Geometry check sheet. Reference: the model listing, model coordinates, mm. A direction names the side the tool comes from. Round coordinates to 2 decimals unless told otherwise and drop trailing zeros. Write each loop counter-clockwise with the first axis right and the second up, starting at its lowest first coordinate (ties: lowest second). Pieces come first, ordered by that corner, then holes. Notation, with made-up numbers: M 19,32 L 70,32 A17 cw 70,52 Z; hole C -6.5,4.5 d10. An arc over 180 degrees is marked long. Use a Markdown table: item, result.
Autodesk Inventor part; units mm, degrees
ref_plane "YZ Plane" through (0, 0, 0) normal (1, 0, 0) x (0, 1, 0)
ref_plane "XZ Plane" through (0, 0, 0) normal (0, 1, 0) x (-1, 0, 0)
ref_plane "XY Plane" through (0, 0, 0) normal (0, 0, 1) x (1, 0, 0)
sketch "Szkic1" plane through (0, 0, 0) normal (0, 0, 1) x (1, 0, 0)
  arc A0 (-1.732, -4.0613) -> (-1.6613, -4.132) centre (0, -2.4) ccw
  arc A1 (0.05, -0.4006) -> (-0.05, -0.4006) centre (0, -2.4) ccw
  arc A2 (-0.05, -0.4006) -> (-0.5703, -0.483) centre (0, -2.4) ccw
  arc A3 (-0.5703, -0.483) -> (-0.6654, -0.5139) centre (0, -2.4) ccw
  arc A4 (-0.6654, -0.5139) -> (-1.1348, -0.7531) centre (0, -2.4) ccw
  arc A5 (-1.1348, -0.7531) -> (-1.2157, -0.8119) centre (0, -2.4) ccw
  arc A6 (-1.2157, -0.8119) -> (-1.5881, -1.1843) centre (0, -2.4) ccw
  arc A7 (-1.5881, -1.1843) -> (-1.6469, -1.2652) centre (0, -2.4) ccw
  arc A8 (-1.6469, -1.2652) -> (-1.8861, -1.7346) centre (0, -2.4) ccw
  arc A9 (-1.8861, -1.7346) -> (-1.917, -1.8297) centre (0, -2.4) ccw
  arc A10 (-1.917, -1.8297) -> (-1.9994, -2.35) centre (0, -2.4) ccw
  arc A11 (-1.9994, -2.35) -> (-1.9994, -2.45) centre (0, -2.4) ccw
  arc A12 (-1.9994, -2.45) -> (-1.917, -2.9703) centre (0, -2.4) ccw
  arc A13 (-1.917, -2.9703) -> (-1.8861, -3.0654) centre (0, -2.4) ccw
  arc A14 (-1.8861, -3.0654) -> (-1.6469, -3.5348) centre (0, -2.4) ccw
  arc A15 (-1.6469, -3.5348) -> (-1.5881, -3.6157) centre (0, -2.4) ccw
  arc A16 (-1.5881, -3.6157) -> (-1.2157, -3.9881) centre (0, -2.4) ccw
  arc A17 (-1.2157, -3.9881) -> (-1.1348, -4.0469) centre (0, -2.4) ccw
  arc A18 (-1.1348, -4.0469) -> (-0.6654, -4.2861) centre (0, -2.4) ccw
  arc A19 (-0.6654, -4.2861) -> (-0.5703, -4.317) centre (0, -2.4) ccw
  arc A20 (-0.5703, -4.317) -> (-0.05, -4.3994) centre (0, -2.4) ccw
  arc A21 (-0.05, -4.3994) -> (0.05, -4.3994) centre (0, -2.4) ccw
  arc A22 (0.05, -4.3994) -> (0.5703, -4.317) centre (0, -2.4) ccw
  arc A23 (0.5703, -4.317) -> (0.6654, -4.2861) centre (0, -2.4) ccw
  arc A24 (0.6654, -4.2861) -> (1.1348, -4.0469) centre (0, -2.4) ccw
  arc A25 (1.1348, -4.0469) -> (1.2157, -3.9881) centre (0, -2.4) ccw
  arc A26 (1.2157, -3.9881) -> (1.5881, -3.6157) centre (0, -2.4) ccw
  arc A27 (1.5881, -3.6157) -> (1.6469, -3.5348) centre (0, -2.4) ccw
  arc A28 (1.6469, -3.5348) -> (1.8861, -3.0654) centre (0, -2.4) ccw
  arc A29 (1.8861, -3.0654) -> (1.917, -2.9703) centre (0, -2.4) ccw
  arc A30 (1.917, -2.9703) -> (1.9994, -2.45) centre (0, -2.4) ccw
  arc A31 (1.9994, -2.45) -> (1.9994, -2.35) centre (0, -2.4) ccw
  arc A32 (1.9994, -2.35) -> (1.917, -1.8297) centre (0, -2.4) ccw
  arc A33 (1.917, -1.8297) -> (1.8861, -1.7346) centre (0, -2.4) ccw
  arc A34 (1.8861, -1.7346) -> (1.6469, -1.2652) centre (0, -2.4) ccw
  arc A35 (1.6469, -1.2652) -> (1.5881, -1.1843) centre (0, -2.4) ccw
  arc A36 (1.5881, -1.1843) -> (1.2157, -0.8119) centre (0, -2.4) ccw
  arc A37 (1.2157, -0.8119) -> (1.1348, -0.7531) centre (0, -2.4) ccw
  arc A38 (1.1348, -0.7531) -> (0.6654, -0.5139) centre (0, -2.4) ccw
  arc A39 (0.6654, -0.5139) -> (0.5703, -0.483) centre (0, -2.4) ccw
  arc A40 (0.5703, -0.483) -> (0.05, -0.4006) centre (0, -2.4) ccw
  circle A41 centre (0, -2.4) radius 1.5065
  circle A42 centre (0, -2.4) radius 2.4
  circle A43 centre (0, -2.4) radius 15
  circle A44 centre (0, -2.4) radius 1.0065
  circle A45 centre (0, -2.4) radius 1.2565
  circle A46 centre (0, -2.4) radius 2.9
  point P0 (0, 0)
  point P1 (-1.6613, -4.132)
  point P2 (-1.732, -4.0613)
  dimension "d0" = 30
  dimension "d3" = 0.25
  dimension "d12" = 0.5
extrude "Wyciągnięcie proste1" add sketch "Szkic1" against normal blind 3 contours A43
extrude "Wyciągnięcie proste2" add sketch "Szkic1" along normal blind 1.5 contours A42 A0 | A40 A39 A38 A37 A36 A35 A34 A33 A32 A31 A30 A29 A28 A27 A26 A25 A24 A23 A22 A21 A20 A19 A18 A17 A16 A15 A14 A13 A12 A11 A10 A9 A8 A7 A6 A5 A4 A3 A2 A1 | A41 | A43 | A45 | A46
sketch "Szkic2" plane through (0, -2.4, 1.5) normal (0, 0, 1) x (1, 0, 0)
  circle A0 centre (0, 0) radius 1.0065
  circle A1 centre (0, 0) radius 3
  circle A2 centre (0, 0) radius 15
  point P0 (0, 2.4)
  dimension "d6" = 6
extrude "Wyciągnięcie proste3" add sketch "Szkic2" along normal blind 2.7 contours A2
sketch "Szkic4" plane through (0, -2.4, -3) normal (0, 0, -1) x (-1, 0, 0)
  arc A0 (6.703, -7.1797) -> (6.021, -7.7605) centre (12.6436, -14.8459) ccw
  arc A1 (9.8735, -5.5514) -> (9.0277, -5.8466) centre (12.6436, -14.8459) ccw
  arc A2 (13.4181, -5.1783) -> (12.5228, -5.1481) centre (12.6436, -14.8459) ccw
  arc A3 (16.8582, -6.1109) -> (16.0342, -5.7593) centre (12.6436, -14.8459) ccw
  arc A4 (19.729, -8.2232) -> (19.0877, -7.5977) centre (12.6436, -14.8459) ccw
  arc A5 (21.6429, -11.23) -> (21.2709, -10.4151) centre (12.6436, -14.8459) ccw
  arc A6 (22.3415, -14.7251) -> (22.2889, -13.8308) centre (12.6436, -14.8459) ccw
  arc A7 (21.7302, -18.2365) -> (22.0043, -17.3836) centre (12.6436, -14.8459) ccw
  arc A8 (19.8918, -21.29) -> (20.4555, -20.5937) centre (12.6436, -14.8459) ccw
  arc A9 (3.9087, -10.6314) -> (5.6223, -12.2259) centre (9.734, -6.0892) ccw
  arc A10 (5.6223, -12.2259) -> (5.4105, -12.8849) centre (12.6436, -14.8459) ccw
  arc A11 (5.4105, -12.8849) -> (3.0888, -13.1827) centre (5.1774, -20.2681) ccw
  arc A12 (3.0888, -13.1827) -> (2.9761, -14.0714) centre (12.6436, -14.8459) ccw
  arc A13 (2.9761, -14.0714) -> (5.1499, -14.9393) centre (6.7672, -7.7316) ccw
  arc A14 (5.1499, -14.9393) -> (5.1905, -15.6303) centre (12.6436, -14.8459) ccw
  arc A15 (5.1905, -15.6303) -> (3.1332, -16.7466) centre (7.6403, -22.5991) ccw
  arc A16 (3.1332, -16.7466) -> (3.3491, -17.616) centre (12.6436, -14.8459) ccw
  arc A17 (3.3491, -17.616) -> (5.6897, -17.64) centre (4.594, -10.3348) ccw
  arc A18 (5.6897, -17.64) -> (5.9772, -18.2697) centre (12.6436, -14.8459) ccw
  arc A19 (5.9772, -18.2697) -> (4.462, -20.0539) centre (10.7789, -23.883) ccw
  arc A20 (4.462, -20.0539) -> (4.9774, -20.7866) centre (12.6436, -14.8459) ccw
  arc A21 (4.9774, -20.7866) -> (7.1686, -19.9634) centre (3.508, -13.5473) ccw
  arc A22 (7.1686, -19.9634) -> (7.6642, -20.4467) centre (12.6436, -14.8459) ccw
  arc A23 (7.6642, -20.4467) -> (6.8958, -22.6577) centre (14.1694, -23.9463) ccw
  arc A24 (6.8958, -22.6577) -> (7.6411, -23.1547) centre (12.6436, -14.8459) ccw
  arc A25 (7.6411, -23.1547) -> (9.387, -21.5956) centre (3.6558, -16.9352) ccw
  arc A26 (9.387, -21.5956) -> (10.0237, -21.8673) centre (12.6436, -14.8459) ccw
  arc A27 (10.0237, -21.8673) -> (10.1059, -24.2066) centre (17.3539, -22.7806) ccw
  arc A28 (10.1059, -24.2066) -> (10.9804, -24.4008) centre (12.6436, -14.8459) ccw
  arc A29 (10.9804, -24.4008) -> (12.0452, -22.3162) centre (5.0175, -20.0409) ccw
  arc A30 (12.0452, -22.3162) -> (12.737, -22.3396) centre (12.6436, -14.8459) ccw
  arc A31 (12.737, -22.3396) -> (13.6588, -24.4912) centre (19.9021, -20.5433) ccw
  arc A32 (13.6588, -24.4912) -> (14.5444, -24.3564) centre (12.6436, -14.8459) ccw
  arc A33 (14.5444, -24.3564) -> (14.7842, -22.028) centre (7.4091, -22.4449) ccw
  arc A34 (14.7842, -22.028) -> (15.4377, -21.7998) centre (12.6436, -14.8459) ccw
  arc A35 (15.4377, -21.7998) -> (17.0745, -23.4732) centre (21.4701, -17.5365) ccw
  arc A36 (17.0745, -23.4732) -> (17.8516, -23.0275) centre (12.6436, -14.8459) ccw
  arc A37 (17.8516, -23.0275) -> (17.2341, -20.7697) centre (10.5077, -23.8227) ccw
  arc A38 (17.2341, -20.7697) -> (17.7611, -20.3209) centre (12.6436, -14.8459) ccw
  arc A39 (17.7611, -20.3209) -> (19.8918, -21.29) centre (21.846, -14.1663) ccw
  arc A40 (20.4555, -20.5937) -> (19.0641, -18.7114) centre (13.8947, -23.9881) ccw
  arc A41 (19.0641, -18.7114) -> (19.3933, -18.1026) centre (12.6436, -14.8459) ccw
  arc A42 (19.3933, -18.1026) -> (21.7302, -18.2365) centre (20.9791, -10.8879) ccw
  arc A43 (22.0043, -17.3836) -> (20.0269, -16.1311) centre (17.1128, -22.9188) ccw
  arc A44 (20.0269, -16.1311) -> (20.114, -15.4444) centre (12.6436, -14.8459) ccw
  arc A45 (20.114, -15.4444) -> (22.3415, -14.7251) centre (18.9865, -8.1441) ccw
  arc A46 (22.2889, -13.8308) -> (19.9926, -13.3772) centre (19.7273, -20.7593) ccw
  arc A47 (19.9926, -13.3772) -> (19.8257, -12.7054) centre (12.6436, -14.8459) ccw
  arc A48 (19.8257, -12.7054) -> (21.6429, -11.23) centre (16.1372, -6.3053) ccw
  arc A49 (21.2709, -10.4151) -> (18.9658, -10.8216) centre (21.3851, -17.801) ccw
  arc A50 (18.9658, -10.8216) -> (18.5675, -10.2554) centre (12.6436, -14.8459) ccw
  arc A51 (18.5675, -10.2554) -> (19.729, -8.2232) centre (12.816, -5.6201) ccw
  arc A52 (19.0877, -7.5977) -> (17.0851, -8.8095) centre (21.8623, -14.4437) ccw
  arc A53 (17.0851, -8.8095) -> (16.5092, -8.4255) centre (12.6436, -14.8459) ccw
  arc A54 (16.5092, -8.4255) -> (16.8582, -6.1109) centre (9.4716, -6.1808) ccw
  arc A55 (16.0342, -5.7593) -> (14.6046, -7.6127) centre (21.0945, -11.1407) ccw
  arc A56 (14.6046, -7.6127) -> (13.9288, -7.4626) centre (12.6436, -14.8459) ccw
  arc A57 (13.9288, -7.4626) -> (13.4181, -5.1783) centre (6.5556, -7.9118) ccw
  arc A58 (12.5228, -5.1481) -> (11.8593, -7.3928) centre (19.1854, -8.3381) ccw
  arc A59 (11.8593, -7.3928) -> (11.1749, -7.4969) centre (12.6436, -14.8459) ccw
  arc A60 (11.1749, -7.4969) -> (9.8735, -5.5514) centre (4.4619, -10.5793) ccw
  arc A61 (9.0277, -5.8466) -> (9.2198, -8.1794) centre (16.3927, -6.4144) ccw
  arc A62 (9.2198, -8.1794) -> (8.6193, -8.5238) centre (12.6436, -14.8459) ccw
  arc A63 (8.6193, -8.5238) -> (6.703, -7.1797) centre (3.4731, -13.823) ccw
  arc A64 (6.021, -7.7605) -> (7.0428, -9.8664) centre (13.0938, -5.6294) ccw
  arc A65 (7.0428, -9.8664) -> (6.6073, -10.4044) centre (12.6436, -14.8459) ccw
  arc A66 (6.6073, -10.4044) -> (4.3348, -9.8434) centre (3.7228, -17.2049) ccw
  arc A67 (4.3348, -9.8434) -> (3.9087, -10.6314) centre (12.6436, -14.8459) ccw
  point P0 (0, 2.4)
  point P1 (0, 0)
extrude "Wyciągnięcie proste5" cut sketch "Szkic4" against normal blind 10 keep common part
properties part number "small-gear"
Item 1: Material ranges on line 1 along Y through (x, z) = (-6.75, -2.5); line 2 along Y through (x, z) = (-6.25, 2.75); line 3 along X through (y, z) = (-9.25, 1.5), recorded low to high. Write a range as from..to.
Outcome:
| item | result |
|---|---|
| line 1 | y = -15.8..-12.62, -11.81..-9.6 |
| line 2 | y = -16.04..-12.66, -10.81..-9.95 |
| line 3 | x = -13.34..-11.95, -10.84..-9.02 |
Item 2: Cross-section at C-C, the plane x = -8. Record the cut outline in (y, z), and give its area (3 significant figures).
Outcome:
| item | result |
|---|---|
| outline | M -15.09,-3 L -10.39,-3 L -10.39,4.2 L -15.09,4.2 Z |
| area | 33.9 mm2 |
Item 3: Cross-section at A-A, the plane z = 2.5. Record the cut outline in (x, y).
Outcome:
| item | result |
|---|---|
| outline | M -13.71,-8.48 A15 ccw -3.82,-16.91 A7.39 ccw -2.98,-16.47 A9.7 ccw -3.09,-15.58 A7.38 ccw -5.41,-15.28 A7.5 ccw -5.62,-14.63 A7.39 ccw -3.91,-13.03 A9.68 ccw -4.33,-12.24 A7.38 ccw -6.61,-12.8 A7.48 ccw -7.04,-12.27 A7.39 ccw -6.02,-10.16 A9.71 ccw -6.7,-9.58 A7.39 ccw -8.62,-10.92 A7.47 ccw -9.22,-10.58 A7.39 ccw -9.03,-8.25 A9.72 ccw -9.87,-7.95 A7.39 ccw -11.17,-9.9 A7.53 ccw -11.86,-9.79 A7.38 ccw -12.52,-7.55 A9.69 ccw -13.42,-7.58 A7.39 ccw Z |
Item 4: Access from +Z, -Z, +X, -X, +Y, -Y to the whole of each face (thin tool, end or side, straight path). Record for faces 4 (the face through (-4.69, -13.886, 0.55)), 5 (the face through (-3.39, -16.7, 0.55)), 6 (the face through (-5.509, -12.437, 0.55)), 7 (the face through (-12.106, -8.628, 0.55)).
Outcome:
| item | result |
|---|---|
| face 4 | +Z, -Z, +X |
| face 5 | +Z, -Z, +X, -Y |
| face 6 | +Z, -Z |
| face 7 | +Z, -Z, +Y |
Item 5: Cross-section at B-B, the plane y = -13.5. Record the cut outline in (x, z).
Outcome:
| item | result |
|---|---|
| outline | M -10.09,-3 L -4.31,-3 L -4.31,4.2 L -10.09,4.2 Z |
Item 6: Mould release check, pull along X, two halves, no side actions. Record for faces 1 (the face through (-3.023, -16.02, 0.55)), 2 (the face through (-13.58, -8.03, 0.55)), 3 (the face through (-7.728, -10.185, 0.55)): +X half, -X half, draft (parallel to the pull), parting line (faces both ways), or undercut.
Outcome:
| item | result |
|---|---|
| face 1 | +X half |
| face 2 | -X half |
| face 3 | undercut |
Item 7: Go/stop test with flat-tipped pins: pin 1 (3 mm diameter, centred on x = -12, z = 2, fed in from -Y); pin 2 (2 mm diameter, centred on x = -12, z = 1, fed in from -Y); pin 3 (1.5 mm diameter, centred on x = -5, z = 0.5, fed in from -Y). Record where each tip stops, or that it passes through.
Outcome:
| item | result |
|---|---|
| pin 1 | stops at y = -13.11 |
| pin 2 | stops at y = -12.6 |
| pin 3 | stops at y = -16.79 |
